Build history of the part. All positions in model axes, mm. A direction names the side the tool comes from. Give positions to 0.01 mm unless a question says otherwise; leave off trailing zeros. Order: outer loops, then holes, each group sorted by start corner. A loop starts at its lowest first (then second) coordinate and runs counter-clockwise, first axis right, second up. Notation, with made-up numbers: M 44,70.5 L 96,70.5 A14 ccw 96,77.5 Z; hole C -37,8 d5. An arc over 180 degrees is marked long. One line per item, written item: value. Start each with the question number.
from build123d import *

# Parameters (mm, degrees)
F0_R     = 7.14375
F1_DEPTH = 6.35
F2_R     = 3.175
F3_DEPTH = 38.1
F4_SIZE  = 0.79375


with BuildPart() as f1:
    # F0 (on Right) → F1 (new body)
    with BuildSketch(Plane.YZ):
        Circle(F0_R)
    extrude(amount=F1_DEPTH)

    # F2 (on face) → F3 (join)
    with BuildSketch(Plane.YZ.offset(6.35)):
        Circle(F2_R)
    extrude(amount=F3_DEPTH)

    # F4
    f4_edges = [f1.edges().sort_by_distance(p)[0] for p in [
        (6.35, -7.14375, 0),
        (0, -7.14375, 0),
        (44.45, -3.175, 0),
    ]]
    chamfer(f4_edges, length=F4_SIZE)


solid = f1.part
1) Slice it at A-A (y = 0). List the corners of the cut face in (x, z) (3 decimals), plus the area to 3 significant figures.
2) Drill centre lines: line 1 (X direction, y = 0, z = 5.25); line 2 (Z direction, x = 12, y = -0.25); line 3 (Z direction, x = 37, y = -1.25). Where is each one in solid material? Low to high.
3) Drop flat-ended pins along their axis: P1, Ø6, axis at x = 20, z = 2.5, coming from the +Y side (3 decimals); P2, Ø5, axis at x = 20, y = -0.5, coming from the +Z side (3 decimals); P3, Ø5, axis at x = 40, z = 1, coming from the -Y side (3 decimals). Give the stop position or say it passes through.
4) Tool access for faces 1 (the cylindrical face through (3.142, -7.137, 0.314)), 2 (the cylindrical face through (24.74, -0.69, -3.1)): list every direction of +Z, -Z, +X, -X, +Y, -Y with a clear straight run to the whole face (end or side of a thin tool).
5) Slice it at B-B (x = 12). List the corners of the cut face in (y, z) (3 decimals).
Results list:
1. outline: M 0,-6.35 L 0.794,-7.144 L 5.556,-7.144 L 6.35,-6.35 L 6.35,-3.175 L 43.656,-3.175 L 44.45,-2.381 L 44.45,2.381 L 43.656,3.175 L 6.35,3.175 L 6.35,6.35 L 5.556,7.144 L 0.794,7.144 L 0,6.35 Z
1. area: 331 mm²
2. line 1: x = 0 to 6.35
2. line 2: z = -3.17 to 3.17
2. line 3: z = -2.92 to 2.92
3. P1: stops at y = 3.175
3. P2: stops at z = 3.175
3. P3: stops at y = -3.175
4. face 1: +X, -X
4. face 2: +X
5. outline: C 0,0 d6.35
